Verification items for the finished model (mm, model axes). A direction names the side the tool comes from. Give positions to 0.01 mm unless a question says otherwise; leave off trailing zeros. Order: outer loops, then holes, each group sorted by start corner. A loop starts at its lowest first (then second) coordinate and runs counter-clockwise, first axis right, second up. Notation, with made-up numbers: (87, 2.25) -> (92, 2.25) arc R19 ccw to (92, 17.25) -> close; hole circle Ø1 at (61, 38.5). An arc over 180 degrees is marked (long way). One line per question, with ' | ' between items. Start each with the question number.
Q1. Mould release check, pull along Y, two halves, no side actions. Record for faces 1 (the flat face through (11.3, 66.5, -6.2)), 2 (the cylindrical face through (13.67, 61.01, 3.03)), 3 (the flat face through (3, 58, -3)): released by +Y, released by -Y, zero draft, split by the parting line, or undercut.
Q2. Section check A-A on z = 0. Record the cut outline in (x, y), plus the area to 3 significant figures.
Q3. Access from +Z, -Z, +X, -X, +Y, -Y to the whole of each face (thin tool, end or side, straight path). Record for faces 4 (the flat face through (11.3, 64.1, 6.2)), 5 (the cylindrical face through (13.67, 66.75, 3.03)), 6 (the cylindrical face through (3.417, 28.594, 0.759)).
Q4. Section check C-C on y = 57. Record the cut outline in (x, z), plus the area to 3 significant figures.
Q5. Material ranges on probe 1 along Y at (x, z) = (5.5, -8.5); probe 2 along Z at (x, y) = (-0.25, 36); probe 3 along Y at (x, z) = (-11.5, 7.75), recorded low to high. Write a range as [from, to].
Q6. Go/stop test with flat-tipped pins: pin 1 (12 mm diameter, centred on x = 7.5, y = 34.5, fed in from +Z); pin 2 (8.5 mm diameter, centred on x = -7, z = 4, fed in from -Y); pin 3 (2 mm diameter, centred on y = 18.5, z = 3.5, fed in from +X); pin 4 (8 mm diameter, centred on y = 27, z = -9, fed in from -X). Record where each tip stops, or that it passes through.
Q7. Section check B-B on x = 0. Record the cut outline in (y, z).
from build123d import *

# Parameters (mm, degrees)
SMUSSO1_SIZE = 1


with BuildPart() as part:
    # Schizzo1 → Rivoluzione1 (revolve)
    with BuildSketch(Plane.XY, mode=Mode.PRIVATE) as rivoluzione1_sk:
        Polygon((-3.5, 0), (0, 0), (0, 68), (-14, 68), (-14, 66.5), (-12.7, 66.5), (-12.7, 64.1), (-14, 64.1), (-14, 58), (-3.5, 58), align=None)
    revolve(rivoluzione1_sk.sketch.rotate(Axis((0, 0, 0), (0, 1, 0)), 270), axis=Axis((0, 0, 0), (0, 1, 0)))

    # Smusso1
    smusso1_edges = [part.edges().sort_by_distance(p)[0] for p in [
        (0, 68, 14),
    ]]
    chamfer(smusso1_edges, length=SMUSSO1_SIZE)


solid = part.part
Filled in:
1) face 1: undercut | face 2: zero draft | face 3: released by -Y
2) outline: (-14, 58) -> (-3.5, 58) -> (-3.5, 0) -> (3.5, 0) -> (3.5, 58) -> (14, 58) -> (14, 64.1) -> (12.7, 64.1) -> (12.7, 66.5) -> (14, 66.5) -> (14, 67) -> (13, 68) -> (-13, 68) -> (-14, 67) -> (-14, 66.5) -> (-12.7, 66.5) -> (-12.7, 64.1) -> (-14, 64.1) -> close | area: 679 mm²
3) face 4: none | face 5: +Y, -Y | face 6: -Y
4) outline: circle Ø7 at (0, 0) | area: 38.5 mm²
5) probe 1: [58, 68] | probe 2: [-3.49, 3.49] | probe 3: [58, 64.1], [66.5, 67.13]
6) pin 1: z = 3.16 | pin 2: y = 58 | pin 3: x = 2.45 | pin 4: through
7) outline: (0, -3.5) -> (58, -3.5) -> (58, -14) -> (64.1, -14) -> (64.1, -12.7) -> (66.5, -12.7) -> (66.5, -14) -> (67, -14) -> (68, -13) -> (68, 13) -> (67, 14) -> (66.5, 14) -> (66.5, 12.7) -> (64.1, 12.7) -> (64.1, 14) -> (58, 14) -> (58, 3.5) -> (0, 3.5) -> close
